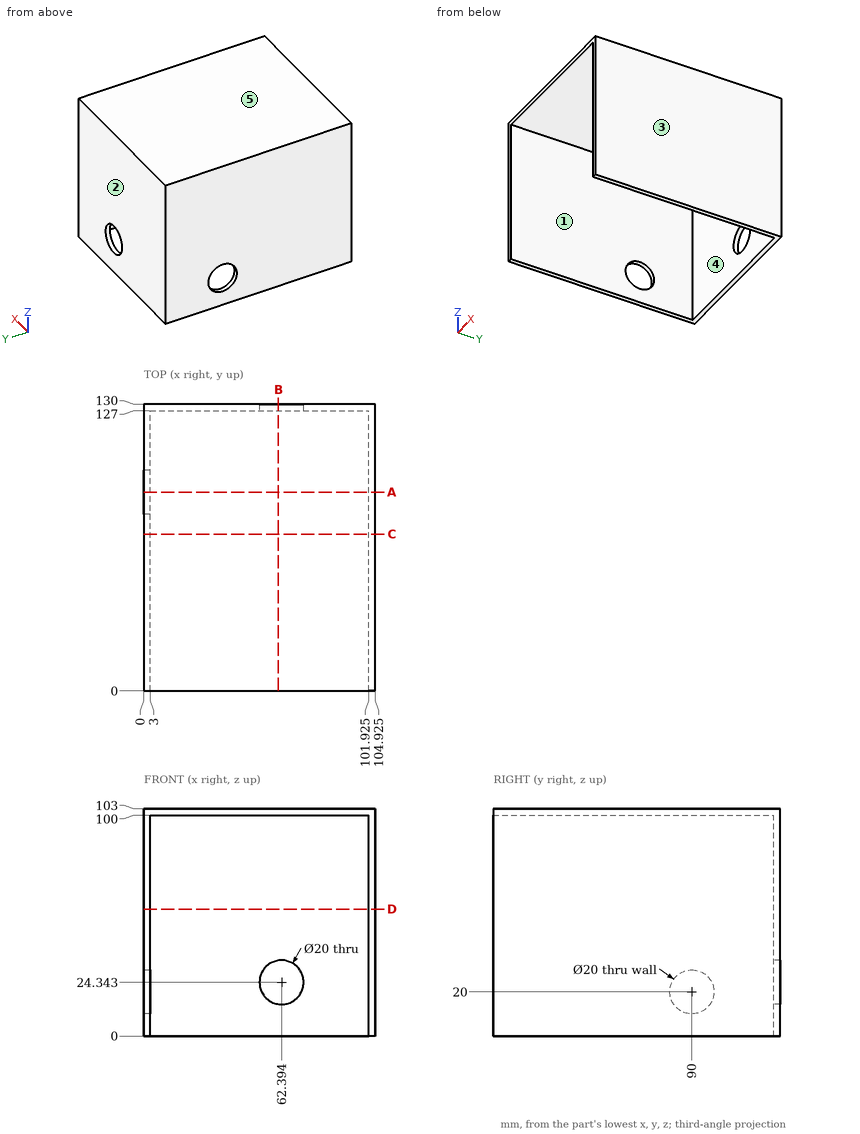
Geometry: see drawing. Coordinates: mm, zero at the bounding-box minimum. A direction names the side the tool comes from. Give positions to 0.01 mm unless a question says otherwise; leave off trailing zeros. Order: outer loops, then holes, each group sorted by start corner. A loop starts at its lowest first (then second) coordinate and runs counter-clockwise, first axis right, second up.
Q1. Set-up query: the marked faces 1 and 2. Return all of +Z, -Z, +X, -X, +Y, -Y with unobstructed straight access to the full face (end or side cutting, diameter ignored); none if empty.
Checked values:
face 1: -Z, -Y
face 2: +Z, -Z, +X, -X, +Y
Q2. Draft query along X for the marked faces 3, 4 and 5. Return one class per face: +X half, -X half, draft (parallel to the pull), parting line (faces both ways), or undercut.
Checked values:
face 3: +X half
face 4: undercut
face 5: draft
Q3. Contact query for a flat-ended pin moving along its axis: pin 1 Ø10 at (x, z) = (33, 90) entering from -Y. Output: stop coordinate, or through.
Checked values:
pin 1: stops at y = 127
Q4. Section D-D on z = 57.5. Output: boundary loops of the cut face in (x, y) (1 decimal), and give its area (3 significant figures).
Checked values:
outline: (0, 0) - (3, 0) - (3, 127) - (101.9, 127) - (101.9, 0) - (104.9, 0) - (104.9, 130) - (0, 130) - close
area: 1,080 mm2
Q5. Section A-A on y = 90. Output: boundary loops of the cut face in (x, z) (1 decimal).
Checked values:
outline: (0, 0) - (3, 0) - (3, 10) - (0, 10) - close; (0, 30) - (3, 30) - (3, 100) - (101.9, 100) - (101.9, 0) - (104.9, 0) - (104.9, 103) - (0, 103) - close
Q6. Section B-B on x = 61. Output: boundary loops of the cut face in (y, z) (1 decimal).
Checked values:
outline: (0, 100) - (127, 100) - (127, 34.2) - (130, 34.2) - (130, 103) - (0, 103) - close; (127, 0) - (130, 0) - (130, 14.4) - (127, 14.4) - close
Q7. Ray query, probe 1 along X at (y, z) = (82, 44) (1 decimal); probe 2 along Y at (x, z) = (2.1, 20); probe 3 along Y at (x, z) = (80, 20.5). Return the intervals inside material, ascending.
Checked values:
probe 1: x = 0 to 3, 101.9 to 104.9
probe 2: y = 0 to 80, 100 to 130
probe 3: y = 127 to 130
Q8. Section C-C on y = 71. Output: boundary loops of the cut face in (x, z) (1 decimal).
Checked values:
outline: (0, 0) - (3, 0) - (3, 100) - (101.9, 100) - (101.9, 0) - (104.9, 0) - (104.9, 103) - (0, 103) - close
